For this review, use the dimensioned drawing (mm, ordinates from the lowest corner) and the shaded views. A direction names the side the tool comes from. Round coordinates to 2 decimals unless told otherwise and drop trailing zeros. Order: outer loops, then holes, each group sorted by start corner. A loop starts at its lowest first (then second) coordinate and runs counter-clockwise, first axis right, second up. Notation, with made-up numbers: (62.5, 77) - (83.5, 77) arc R19 ccw to (83.5, 99) - close; hole circle Ø1 at (37.25, 79). An arc over 180 degrees is marked (long way). Use CSV: the item, a comma, the result in double quotes. Start each with the question number.
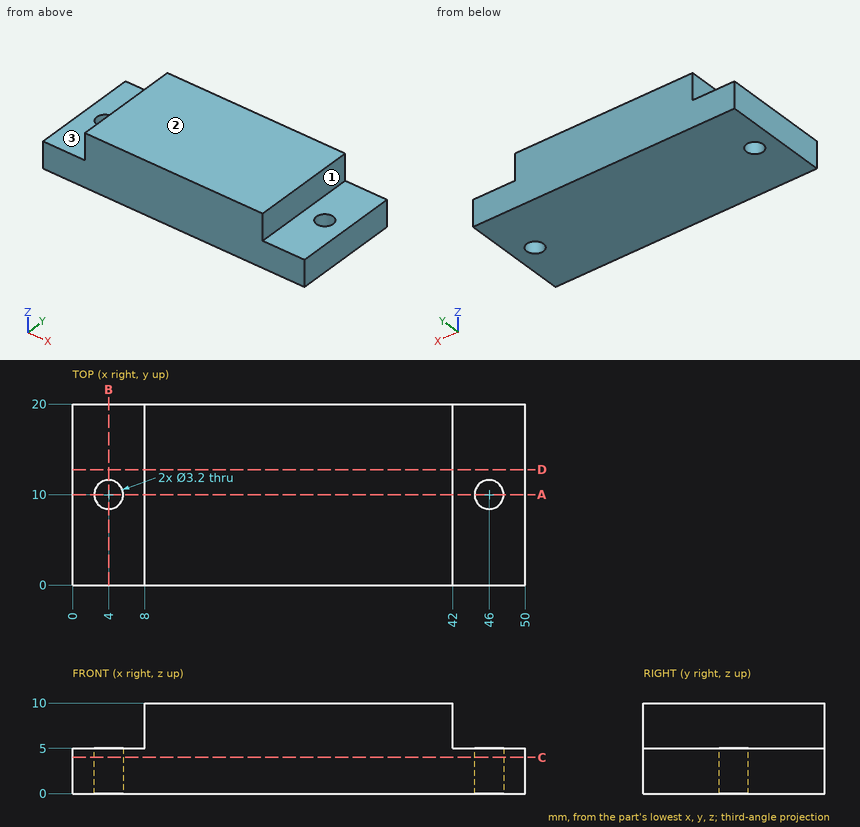
Q1. Take a section at B-B (x = 4). State the section outline as (y, z) points, plus the area to 3 significant figures.
Q2. Clearance check with flat-ended pins moving along their axes: pin 1 (4 mm diameter, centred on x = 5, y = 14, fed in from +Z); pin 2 (4 mm diameter, centred on y = 7, z = 7.5, fed in from +X); pin 3 (2.5 mm diameter, centred on y = 6.5, z = 7.5, fed in from -X); pin 4 (1.9 mm diameter, centred on x = 4, y = 10, fed in from -Z). State where each tip first meets the part, or that it passes through.
Q3. Take a section at C-C (z = 4). State the section outline as (x, y) points, plus the area to 3 significant figures.
Q4. For L1, parallel to Y at x = 4, z = 3.5; L2, parallel to X at y = 10.5, z = 2.5; L3, parallel to X at y = 3.25, z = 8.75, list the stretches that pass through material, from the lowest coordinate up. Write a range as [from, to].
Q5. Take a section at A-A (y = 10). State the section outline as (x, z) points, plus the area to 3 significant figures.
Q6. Tool access review of the marked faces 1, 2 and 3: name each direction out of +Z, -Z, +X, -X, +Y, -Y from which nothing blocks a thin tool from reaching the whole face with its end or side.
Q7. Take a section at D-D (y = 12.75). State the section outline as (x, z) points, plus the area to 3 significant figures.
Findings below:
1,outline,"(0, 0) - (8.4, 0) - (8.4, 5) - (0, 5) - close; (11.6, 0) - (20, 0) - (20, 5) - (11.6, 5) - close"
1,area,"84.0 mm^2"
2,pin 1,"stops at z = 5"
2,pin 2,"stops at x = 42"
2,pin 3,"stops at x = 8"
2,pin 4,"passes through"
3,outline,"(0, 0) - (50, 0) - (50, 20) - (0, 20) - close; hole circle Ø3.2 at (4, 10); hole circle Ø3.2 at (46, 10)"
3,area,"984 mm^2"
4,L1,"y = [0, 8.4], [11.6, 20]"
4,L2,"x = [0, 2.48], [5.52, 44.48], [47.52, 50]"
4,L3,"x = [8, 42]"
5,outline,"(0, 0) - (2.4, 0) - (2.4, 5) - (0, 5) - close; (5.6, 0) - (44.4, 0) - (44.4, 5) - (42, 5) - (42, 10) - (8, 10) - (8, 5) - (5.6, 5) - close; (47.6, 0) - (50, 0) - (50, 5) - (47.6, 5) - close"
5,area,"388 mm^2"
6,face 1,"+Z, +X, +Y, -Y"
6,face 2,"+Z, +X, -X, +Y, -Y"
6,face 3,"+Z, -X, +Y, -Y"
7,outline,"(0, 0) - (50, 0) - (50, 5) - (42, 5) - (42, 10) - (8, 10) - (8, 5) - (0, 5) - close"
7,area,"420 mm^2"
